Input: part model. Units: mm. Frame: model coordinates. Round coordinates to 2 decimals unless told otherwise and drop trailing zeros. Loops run counter-clockwise (first coordinate to the right, second up) from the corner with the lowest first, then second, coordinate; pieces in that order, holes last.
(1) Line query: line 1 (X direction, y = -1.5, z = 0.55); line 2 (X direction, y = 0.5, z = 0.2); line 3 (X direction, y = -0.25, z = 0.4). Output: solid intervals per line, ascending.
(2) First-contact query: pin 1 Ø2.5 at (x, y) = (0.09, 0.66) entering from -Z. Flat tip, straight axial feed; report the tip coordinate or a pass-through.
(3) Cut plane B-B, the plane x = -11. Output: boundary loops of the cut face in (y, z), and give its area (3 significant figures).
(4) Cut plane C-C, the plane x = 10.5. Output: boundary loops of the cut face in (y, z).
(5) Cut plane A-A, the plane z = 0.4. Output: boundary loops of the cut face in (x, y), and give its area (3 significant figures).
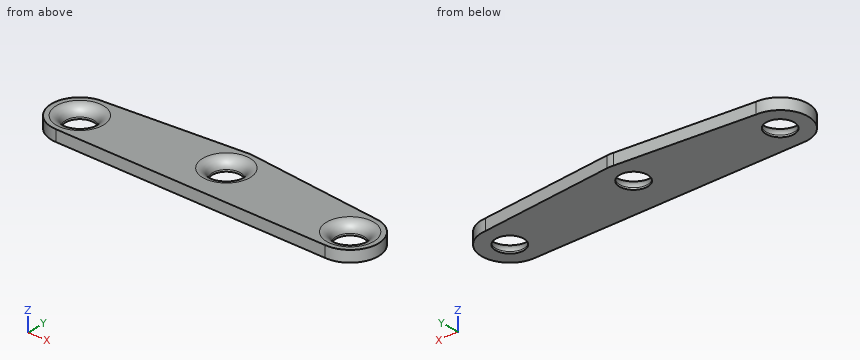
from build123d import *

# Parameters (mm, degrees)
SKETCH_1_R        = 3
SKETCH_1_R_2      = 1.5
EXTRUDE_1_DEPTH   = 1.2
EXTRUDE_1_2_DEPTH = 1.2
EXTRUDE_1_3_DEPTH = 1.2
EXTRUDE_START     = -1.2
EXTRUDE_6_DEPTH   = 1.2
FILLET_1_R        = 1


# Read off the part's stored shape, not the designer's step: the extrude step
with BuildPart() as part:
    # Sketch 1 → Extrude 1 (new body)
    with BuildSketch(Plane.XY):
        with Locations((-14.609483562, -0.654127434)):
            Circle(SKETCH_1_R)
        with Locations((-14.609483562, -0.654127434)):
            Circle(SKETCH_1_R_2, mode=Mode.SUBTRACT)
    extrude(amount=EXTRUDE_1_DEPTH)



with BuildPart() as body_2:
    # Sketch 1 → Extrude 1 2 (new body)
    with BuildSketch(Plane.XY):
        with Locations((0.085103447, 0.656172203)):
            Circle(SKETCH_1_R)
        with Locations((0.085103447, 0.656172203)):
            Circle(SKETCH_1_R_2, mode=Mode.SUBTRACT)
    extrude(amount=EXTRUDE_1_2_DEPTH)


with BuildPart() as body_3:
    # Sketch 1 → Extrude 1 3 (new body)
    with BuildSketch(Plane.XY):
        with Locations((14.609483562, -0.656172203)):
            Circle(SKETCH_1_R)
        with Locations((14.609483562, -0.656172203)):
            Circle(SKETCH_1_R_2, mode=Mode.SUBTRACT)
    extrude(amount=EXTRUDE_1_3_DEPTH)


with BuildPart() as part_1:
    add(part.part)

    add(body_2.part)  # Extrude 6 merges body 2

    add(body_3.part)  # Extrude 6 merges body 3
    # Extrude 6 outline → Extrude 6 (add)
    with BuildSketch(Plane.XY.offset(1.2).offset(EXTRUDE_START)):
        with BuildLine():
            Line((-0.357791462, 3.62329945), (-14.609483562, 2.345872566))
            ThreePointArc((-14.609483562, 2.345872566), (-11.609512533, -0.640943153), (-14.583115254, -3.65401155))
            Line((-14.583115254, -3.65401155), (14.52155751, -3.654883428))
            ThreePointArc((14.52155751, -3.654883428), (11.609805773, -0.612204455), (14.609483562, 2.343827797))
            Line((14.609483562, 2.343827797), (0.357607149, 3.64377019))
            ThreePointArc((0.357607149, 3.64377019), (0.170911685, -2.34260037), (-0.357791462, 3.62329945))
        make_face()
    extrude(amount=EXTRUDE_6_DEPTH)

    # Fillet 1
    fillet_1_edges = [part_1.edges().sort_by_distance(p)[0] for p in [
        (-1.414896553, 0.656172203, 1.2),
        (13.109483562, -0.656172203, 1.2),
        (-16.109483562, -0.654127434, 1.2),
    ]]
    fillet(fillet_1_edges, radius=FILLET_1_R)


solid = part_1.part
Reported:
1. line 1: x = -17.49 to -15.92, -13.29 to 13.29, 15.93 to 17.49
1. line 2: x = -17.38 to -15.57, -13.65 to -1.41, 1.58 to 13.65, 15.57 to 17.38
1. line 3: x = -17.58 to -16.07, -13.14 to -1.14, 1.31 to 13.14, 16.07 to 17.58
2. pin 1: passes through
3. outline: (-3.65, 0) - (2.67, 0) - (2.67, 1.2) - (-3.65, 1.2) - close
3. area: 7.59 mm2
4. outline: (-3.65, 0) - (2.72, 0) - (2.72, 1.2) - (-3.65, 1.2) - close
5. outline: (-14.61, 2.35) arc R3 ccw (long way) to (-14.58, -3.65) - (14.52, -3.65) arc R3 ccw (long way) to (14.61, 2.34) - (0.36, 3.64) arc R3 ccw to (-0.36, 3.62) - close; hole circle Ø3.04 at (-14.61, -0.65); hole circle Ø3.04 at (0.09, 0.66); hole circle Ø3.04 at (14.61, -0.66)
5. area: 201 mm2
